Verification items for the finished model (mm, model axes). A direction names the side the tool comes from. Coordinates: 2 decimals unless noted, no trailing zeros. Write each loop counter-clockwise with the first axis right and the second up, starting at its lowest first coordinate (ties: lowest second). Pieces come first, ordered by that corner, then holes. Notation, with made-up numbers: (-11, 14) -> (35, 14) arc R27 ccw to (35, 43) -> close; hole circle Ø8 at (34.25, 9.25). An arc over 180 degrees is marked (long way). Answer in a Markdown table with one row per item.
```python
from build123d import *

# Parameters (mm, degrees)
F3_DEPTH = 30
F4_DEPTH = 8
F5_R     = 1.5


# Not quite as in the source:
# - ends of sketch curves that miss each other by under 0.0002 mm in the source are joined


with BuildPart() as f3:
    # F0 (on Top) → F3 (new body)
    with BuildSketch(Plane.XY):
        with BuildLine():
            Line((2.7344355629, 17), (0, 17))
            Line((0, 17), (-2.7344355629, 17))
            ThreePointArc((-2.7344355629, 17), (-7.9821831045, 14.6326182171), (-9.6803811114, 9.1317568064))
            Line((-9.6803811114, 9.1317568064), (-8.6803809552, 1.131756826))
            ThreePointArc((-8.6803809552, 1.131756826), (-6.3670534302, -3.2477471454), (-1.7344355629, -4.9999998862))
            Line((-1.7344355629, -4.9999998862), (0, -4.9999998882))
            Line((0, -4.9999998882), (1.7344355629, -5))
            ThreePointArc((1.7344355629, -5), (6.3670535056, -3.2477472307), (8.6803806999, 1.1317568579))
            Line((8.6803806999, 1.1317568579), (9.6803806999, 9.1317568579))
            ThreePointArc((9.6803806999, 9.1317568579), (7.9821826424, 14.6326178092), (2.7344355629, 17))
        make_face()
        with BuildLine():
            Line((1.7344355629, 0), (0, 0))
            Line((0, 0), (-1.7344355629, 0))
            ThreePointArc((-1.7344355629, 0), (-3.0580406894, 0.5006436484), (-3.7189913164, 1.7519305308))
            Line((-3.7189913164, 1.7519305308), (-4.7189913164, 9.7519305308))
            ThreePointArc((-4.7189913164, 9.7519305308), (-4.2337919146, 11.3236051265), (-2.7344355629, 12))
            Line((-2.7344355629, 12), (0, 12))
            Line((0, 12), (2.7344355629, 12))
            ThreePointArc((2.7344355629, 12), (4.2337919146, 11.3236051265), (4.7189913164, 9.7519305308))
            Line((4.7189913164, 9.7519305308), (3.7189913164, 1.7519305308))
            ThreePointArc((3.7189913164, 1.7519305308), (3.0580406894, 0.5006436484), (1.7344355629, 0))
        make_face(mode=Mode.SUBTRACT)
        with BuildLine():
            Line((-1.7344355629, 0), (0, 0))
            Line((0, 0), (0, 3))
            ThreePointArc((0, 3), (-3, 6), (0, 9))
            Line((0, 9), (0, 12))
            Line((0, 12), (-2.7344355629, 12))
            ThreePointArc((-2.7344355629, 12), (-4.2337919146, 11.3236051265), (-4.7189913164, 9.7519305308))
            Line((-4.7189913164, 9.7519305308), (-3.7189913164, 1.7519305308))
            ThreePointArc((-3.7189913164, 1.7519305308), (-3.0580406894, 0.5006436484), (-1.7344355629, 0))
        make_face()
        with BuildLine():
            Line((0, 3), (0, 0))
            Line((0, 0), (1.7344355629, 0))
            ThreePointArc((1.7344355629, 0), (3.0580406894, 0.5006436484), (3.7189913164, 1.7519305308))
            Line((3.7189913164, 1.7519305308), (4.7189913164, 9.7519305308))
            ThreePointArc((4.7189913164, 9.7519305308), (4.2337919146, 11.3236051265), (2.7344355629, 12))
            Line((2.7344355629, 12), (0, 12))
            Line((0, 12), (0, 9))
            ThreePointArc((0, 9), (2.1213203436, 8.1213203436), (3, 6))
            ThreePointArc((3, 6), (2.1213203436, 3.8786796564), (0, 3))
        make_face()
    extrude(amount=F3_DEPTH)

    # F2 (on offset) → F4 (cut)
    with BuildSketch(Plane.XY.offset(30)):
        with BuildLine():
            ThreePointArc((-3.7189913164, 1.7519305308), (-3.0580406894, 0.5006436484), (-1.7344355629, 0))
            Line((-1.7344355629, 0), (0, 0))
            Line((0, 0), (0, 3))
            ThreePointArc((0, 3), (-3, 6), (0, 9))
            Line((0, 9), (0, 12))
            Line((0, 12), (-2.7344355629, 12))
            ThreePointArc((-2.7344355629, 12), (-4.2337919146, 11.3236051265), (-4.7189913164, 9.7519305308))
            Line((-4.7189913164, 9.7519305308), (-3.7189913164, 1.7519305308))
        make_face()
        with BuildLine():
            Line((0, 3), (0, 0))
            Line((0, 0), (1.7344355629, 0))
            ThreePointArc((1.7344355629, 0), (3.0580406894, 0.5006436484), (3.7189913164, 1.7519305308))
            Line((3.7189913164, 1.7519305308), (4.7189913164, 9.7519305308))
            ThreePointArc((4.7189913164, 9.7519305308), (4.2337919146, 11.3236051265), (2.7344355629, 12))
            Line((2.7344355629, 12), (0, 12))
            Line((0, 12), (0, 9))
            ThreePointArc((0, 9), (3, 6), (0, 3))
        make_face()
    extrude(amount=-F4_DEPTH, mode=Mode.SUBTRACT)

    # F5
    f5_edges = [f3.edges().sort_by_distance(p)[0] for p in [
        (-4.233792, 11.323605, 22),
        (-4.218991, 5.751931, 22),
    ]]
    fillet(f5_edges, radius=F5_R)


solid = f3.part
```
1. Sectioned sample at A-A, the plane z = 2.5. Record the cut outline in (x, y), and give its area (3 significant figures).
Findings below:
| item | result |
|---|---|
| outline | (-9.68, 9.13) -> (-8.68, 1.13) arc R7 ccw to (-1.73, -5) -> (1.73, -5) arc R7 ccw to (8.68, 1.13) -> (9.68, 9.13) arc R7 ccw to (2.73, 17) -> (-2.73, 17) arc R7 ccw to start; hole circle Ø6 at (0, 6) |
| area | 337 mm² |
2. Material ranges on probe 1 along X at (y, z) = (3.25, 5); probe 2 along X at (y, z) = (7.5, 20.5); probe 3 along Y at (x, z) = (-1.5, 21.5), recorded low to high. Write a range as from..to.
Findings below:
| item | result |
|---|---|
| probe 1 | x = -8.95..-1.2, 1.2..8.95 |
| probe 2 | x = -9.48..-2.6, 2.6..9.48 |
| probe 3 | y = -5..3.4, 8.6..17 |
3. Sectioned sample at D-D, the plane x = -6.25. Record the cut outline in (y, z).
Findings below:
| item | result |
|---|---|
| outline | (-3.35, 0) -> (16.05, 0) -> (16.05, 30) -> (-3.35, 30) -> close |
4. Sectioned sample at B-B, the plane x = 0.5. Record the cut outline in (y, z), and give its area (3 significant figures).
Findings below:
| item | result |
|---|---|
| outline | (-5, 0) -> (3.04, 0) -> (3.04, 22) -> (1.5, 22) arc R1.5 cw to (0, 23.5) -> (0, 30) -> (-5, 30) -> close; (8.96, 0) -> (17, 0) -> (17, 30) -> (12, 30) -> (12, 23.5) arc R1.5 cw to (10.5, 22) -> (8.96, 22) -> close |
| area | 435 mm² |
5. Go/stop test with flat-tipped pins: pin 1 (1.5 mm diameter, centred on x = 1, y = 3.5, fed in from +Z); pin 2 (1 mm diameter, centred on y = 13, z = 24.5, fed in from +X); pin 3 (6 mm diameter, centred on y = 5.5, z = 7, fed in from +X). Record where each tip stops, or that it passes through.
Findings below:
| item | result |
|---|---|
| pin 1 | stops at z = 22 |
| pin 2 | stops at x = 9.27 |
| pin 3 | stops at x = 9.6 |
6. Access from +Z, -Z, +X, -X, +Y, -Y to the whole of each face (thin tool, end or side, straight path). Record for faces 1 (the face through (0, 12, 27)), 2 (the face through (-4.5, 6.2, 30)).
Findings below:
| item | result |
|---|---|
| face 1 | +Z |
| face 2 | +Z, +X, -X, +Y, -Y |
7. Sectioned sample at C-C, the plane z = 27. Record the cut outline in (x, y).
Findings below:
| item | result |
|---|---|
| outline | (-9.68, 9.13) -> (-8.68, 1.13) arc R7 ccw to (-1.73, -5) -> (1.73, -5) arc R7 ccw to (8.68, 1.13) -> (9.68, 9.13) arc R7 ccw to (2.73, 17) -> (-2.73, 17) arc R7 ccw to start; hole (-4.72, 9.75) -> (-3.72, 1.75) arc R2 ccw to (-1.73, 0) -> (1.73, 0) arc R2 ccw to (3.72, 1.75) -> (4.72, 9.75) arc R2 ccw to (2.73, 12) -> (-2.73, 12) arc R2 ccw to start |
8. Release check for a two-part mould opening along Y. For faces 3 (the face through (3.5, 3.1, 22.5)), 4 (the face through (0, 17, 15)), 5 (the face through (2, 9, 0)), 6 (the face through (6.314, -3.294, 14.79)) record: released by +Y, released by -Y, zero draft, split by the parting line, or undercut.
Findings below:
| item | result |
|---|---|
| face 3 | undercut |
| face 4 | released by +Y |
| face 5 | zero draft |
| face 6 | released by -Y |
